```python
from build123d import *

# Parameters (mm, degrees)
SKETCH_1_W          = 51.55
SKETCH_1_H          = 70.5
SKETCH_1_R          = 1.3
EXTRUDE_1_DEPTH     = 4
SKETCH_2_W          = 51.55
SKETCH_2_H          = 70.5
EXTRUDE_2_DEPTH     = 17.6
SKETCH_4_W          = 47.55
SKETCH_4_H          = 8
CUT_EXTRUDE_1_DEPTH = 12
SKETCH_6_W          = 57.55
SKETCH_6_H          = 15.6
CUT_EXTRUDE_3_DEPTH = 2.2
SKETCH_7_W          = 8
SKETCH_7_H          = 10.60647
CUT_EXTRUDE_4_DEPTH = 2
SKETCH_8_W          = 26
SKETCH_8_H          = 3
CUT_EXTRUDE_5_DEPTH = 83


with BuildPart() as part:
    # 草图1 → 凸台-拉伸1 (new body)
    with BuildSketch(Plane(origin=(0, 0, 0), x_dir=(1, 0, 0), z_dir=(0, 1, 0))):
        Rectangle(SKETCH_1_W, SKETCH_1_H)
        with Locations(Location((-20.3835, 31.1785, 0), (0, 0, 270))):
            Circle(SKETCH_1_R, mode=Mode.SUBTRACT)
        with Locations(Location((20.3835, 31.1785, 0), (0, 0, 90))):
            Circle(SKETCH_1_R, mode=Mode.SUBTRACT)
        with Locations(Location((20.3835, -31.1785, 0), (0, 0, 270))):
            Circle(SKETCH_1_R, mode=Mode.SUBTRACT)
        with Locations(Location((-20.3835, -31.1785, 0), (0, 0, 90))):
            Circle(SKETCH_1_R, mode=Mode.SUBTRACT)
    extrude(amount=EXTRUDE_1_DEPTH)

    # 草图2 → 凸台-拉伸2 (add)
    with BuildSketch(Plane.XZ):
        with BuildLine():
            Line((-23.775, 43.25), (23.775, 43.25))
            ThreePointArc((23.775, 43.25), (30.846067812, 40.321067812), (33.775, 33.25))
            Line((33.775, 33.25), (33.775, -33.25))
            ThreePointArc((33.775, -33.25), (30.846067812, -40.321067812), (23.775, -43.25))
            Line((23.775, -43.25), (-23.775, -43.25))
            ThreePointArc((-23.775, -43.25), (-30.846067812, -40.321067812), (-33.775, -33.25))
            Line((-33.775, -33.25), (-33.775, 33.25))
            ThreePointArc((-33.775, 33.25), (-30.846067812, 40.321067812), (-23.775, 43.25))
        make_face()
        Rectangle(SKETCH_2_W, SKETCH_2_H, mode=Mode.SUBTRACT)
    extrude(amount=-EXTRUDE_2_DEPTH)

    # 草图4 → 切除-拉伸1 (cut)
    with BuildSketch(Plane(origin=(0, 17.6, 0), x_dir=(1, 0, 0), z_dir=(0, 1, 0))):
        with Locations((0, -39.25)):
            Rectangle(SKETCH_4_W, SKETCH_4_H)
    extrude(amount=-CUT_EXTRUDE_1_DEPTH, mode=Mode.SUBTRACT)

    # 草图6 → 切除-拉伸3 (cut)
    with BuildSketch(Plane(origin=(0, 0, 38.05), x_dir=(-1, 0, 0), z_dir=(0, 0, -1))):
        with Locations((-5, 9.8)):
            Rectangle(SKETCH_6_W, SKETCH_6_H)
    extrude(amount=-CUT_EXTRUDE_3_DEPTH, mode=Mode.SUBTRACT)

    # 草图7 → 切除-拉伸4 (cut)
    with BuildSketch(Plane(origin=(0, 17.6, 0), x_dir=(1, 0, 0), z_dir=(0, 1, 0))):
        with Locations((-29.775, 16.673805)):
            Rectangle(SKETCH_7_W, SKETCH_7_H)
    extrude(amount=-CUT_EXTRUDE_4_DEPTH, mode=Mode.SUBTRACT)

    # 草图8 → 切除-拉伸5 (cut)
    with BuildSketch(Plane.ZY.offset(33.775)):
        with Locations((-11.25, 7.6)):
            Rectangle(SKETCH_8_W, SKETCH_8_H)
    extrude(amount=-CUT_EXTRUDE_5_DEPTH, mode=Mode.SUBTRACT)


solid = part.part
```
The listing builds one solid part. Answer for the finished solid, in the listing's coordinates (mm). A direction names the side the tool comes from. Give positions to 0.01 mm unless a question says otherwise; leave off trailing zeros. Order: outer loops, then holes, each group sorted by start corner. A loop starts at its lowest first (then second) coordinate and runs counter-clockwise, first axis right, second up. Notation, with made-up numbers: (-10, -13) -> (2, -13) arc R17 ccw to (2, 15) -> close; hole circle Ø1 at (55, -7). An arc over 180 degrees is marked (long way). One line per item, written item: value.
1) Find section D-D, the plane y = 7.25. Determine the outline of the cut face in (x, z) (3 decimals), plus the area to 3 significant figures.
Reported:
outline: (-33.775, -33.25) arc R10 ccw to (-23.775, -43.25) -> (23.775, -43.25) arc R10 ccw to (33.775, -33.25) -> (33.775, -24.25) -> (25.775, -24.25) -> (25.775, -35.25) -> (-25.775, -35.25) -> (-25.775, -24.25) -> (-33.775, -24.25) -> close; (-33.775, 1.75) -> (-25.775, 1.75) -> (-25.775, 35.25) -> (-23.775, 35.25) -> (-23.775, 43.25) arc R10 ccw to (-33.775, 33.25) -> close; (23.775, 35.25) -> (25.775, 35.25) -> (25.775, 1.75) -> (33.775, 1.75) -> (33.775, 33.25) arc R10 ccw to (32.548, 38.05) -> (23.775, 38.05) -> close; (23.775, 40.25) -> (30.916, 40.25) arc R10 ccw to (23.775, 43.25) -> close
area: 1,310 mm^2
2) Find section C-C, the plane z = -16. Determine the outline of the cut face in (x, y) (3 decimals).
Reported:
outline: (-33.775, 0) -> (33.775, 0) -> (33.775, 6.1) -> (25.775, 6.1) -> (25.775, 4) -> (-25.775, 4) -> (-25.775, 6.1) -> (-33.775, 6.1) -> close; (-33.775, 9.1) -> (-25.775, 9.1) -> (-25.775, 15.6) -> (-33.775, 15.6) -> close; (25.775, 9.1) -> (33.775, 9.1) -> (33.775, 17.6) -> (25.775, 17.6) -> close
3) Find the intervals of material crossed by line 1 (X direction, y = 7.5, z = 18) (3 decimals); line 2 (Z direction, x = -12.5, y = 3.5); line 3 (Y direction, x = -23.5, z = -20.5), in increasing order.
Reported:
line 1: x = -33.775 to -25.775, 25.775 to 33.775
line 2: z = -43.25 to 38.05, 40.25 to 43.25
line 3: y = 0 to 4
4) Find section A-A, the plane y = 13. Determine the outline of the cut face in (x, z) (3 decimals).
Reported:
outline: (-33.775, -33.25) arc R10 ccw to (-23.775, -43.25) -> (23.775, -43.25) arc R10 ccw to (33.775, -33.25) -> (33.775, 33.25) arc R10 ccw to (32.548, 38.05) -> (23.775, 38.05) -> (23.775, 35.25) -> (25.775, 35.25) -> (25.775, -35.25) -> (-25.775, -35.25) -> (-25.775, 35.25) -> (-23.775, 35.25) -> (-23.775, 43.25) arc R10 ccw to (-33.775, 33.25) -> close; (23.775, 40.25) -> (30.916, 40.25) arc R10 ccw to (23.775, 43.25) -> close
5) A tool of negligible diameter and unlimited length cuts with its end or side. For faces 1 (the flat face through (5, 2, 39)), 2 (the flat face through (-25.775, 11, 0)), 3 (the flat face through (-30, 15.6, -17)), from which of +Z, -Z, +X, -X, +Y, -Y can it reach the whole face along a straight path? Write none if from no direction.
Reported:
face 1: +X, +Y
face 2: +Y
face 3: -X, +Y
6) Determine the mould class of faces 4 (the flat face through (0, 9, -43.25)), 5 (the flat face through (-30, 17.6, 16)), 6 (the flat face through (30, 8, 1.75)) for opening direction Z: pulls with the +Z half, pulls with the -Z half, needs draft (parallel to the pull), parting line crosses it, or undercut.
Reported:
face 4: pulls with the -Z half
face 5: needs draft
face 6: undercut
7) Find section B-B, the plane x = 2. Determine the outline of the cut face in (y, z), plus the area to 3 significant figures.
Reported:
outline: (0, -43.25) -> (17.6, -43.25) -> (17.6, -35.25) -> (4, -35.25) -> (4, 35.25) -> (5.6, 35.25) -> (5.6, 38.05) -> (2, 38.05) -> (2, 40.25) -> (5.6, 40.25) -> (5.6, 43.25) -> (0, 43.25) -> close
area: 460 mm^2
8) Flat-ended cylindrical pins translate along their axes: P1, Ø2, axis at x = -12.5, z = 9, coming from the -Y side; P2, Ø1.6, axis at x = -20.38, z = -31.18, coming from the -Y side; P3, Ø1, axis at x = -1, y = 7.5, coming from the +Z side; P4, Ø3, axis at x = 20.38, z = 31.18, coming from the +Y side. Find the tip coordinate at first contact, or state that the pin passes through.
Reported:
P1: stops at y = 0
P2: passes through
P3: stops at z = -35.25
P4: stops at y = 4
